Job drawing, mm, ordinate dimensions from the low corner. One solid piece. A direction names the side the tool comes from. Coordinates: 2 decimals unless noted, no trailing zeros. Write each loop counter-clockwise with the first axis right and the second up, starting at its lowest first coordinate (ties: lowest second). Pieces come first, ordered by that corner, then holes. Notation, with made-up numbers: (88, -13.75) - (115, -13.75) arc R26 ccw to (115, 2.25) - close; hole circle Ø3 at (31.25, -23). An arc over 180 degrees is marked (long way). Put each result on its own line as item: value. Start each with the question number.
1. Saw through at B-B, the plane y = 0.5. Write the cut outline in (x, z).
2. Drill centre lines: L1, parallel to Z at x = 1, y = 2; L2, parallel to Y at x = 4.5, z = 4; L3, parallel to Y at x = 4.5, z = 2.5. Where is each one in solid material? Low to high. Write a range as from..to.
3. Saw through at C-C, the plane x = 6.5. Write the cut outline in (y, z).
4. Pull direction Z, two halves, no side cores. Call the marked faces 3, 4, 5 and 6: released by +Z, released by -Z, zero draft, split by the parting line, or undercut.
5. Which spindle directions (+Z, -Z, +X, -X, +Y, -Y) get a long thin tool onto all of the face, cutting with end or side? Do the marked faces 1 and 2. Say none if no direction does.
6. Saw through at A-A, the plane x = 4.5. Write the cut outline in (y, z).
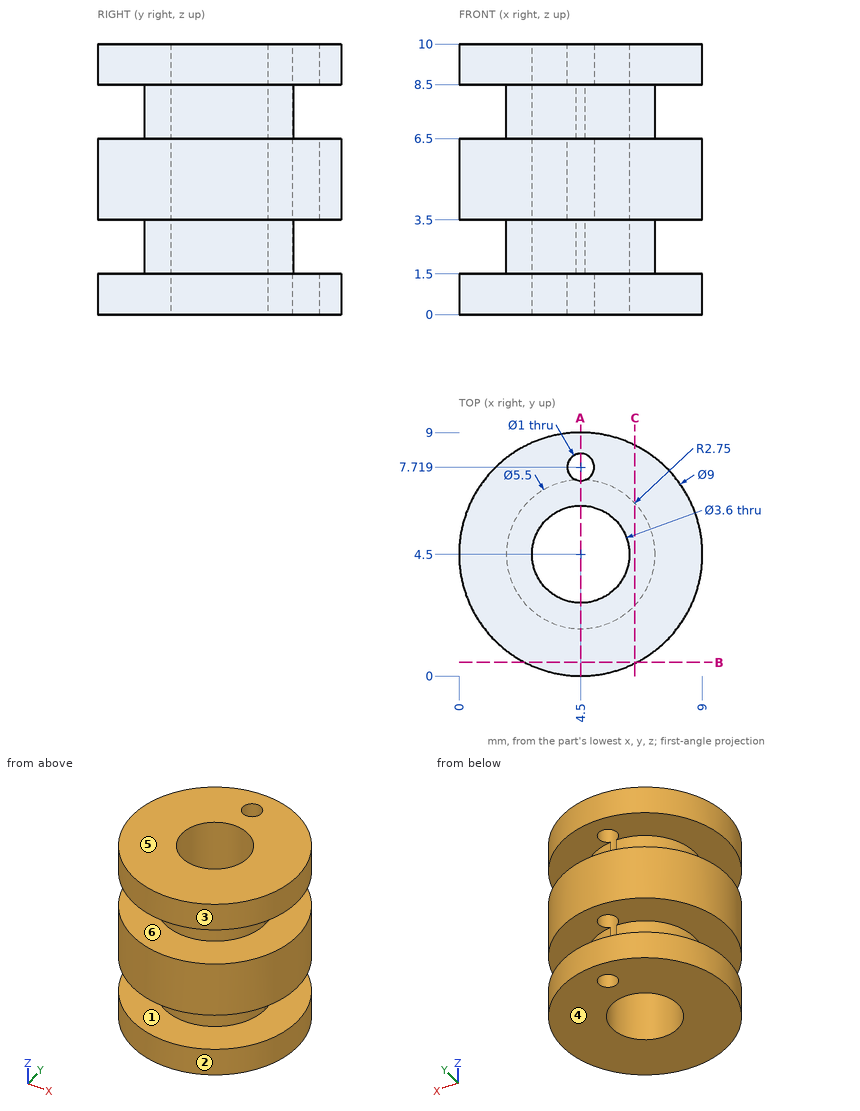
Final values:
1. outline: (2.44, 0) - (6.56, 0) - (6.56, 1.5) - (2.44, 1.5) - close; (2.44, 3.5) - (6.56, 3.5) - (6.56, 6.5) - (2.44, 6.5) - close; (2.44, 8.5) - (6.56, 8.5) - (6.56, 10) - (2.44, 10) - close
2. L1: z = 0..1.5, 3.5..6.5, 8.5..10
2. L2: y = 0..2.7, 6.3..7.22, 8.22..9
2. L3: y = 1.75..2.7, 6.3..7.22
3. outline: (0.47, 0) - (8.53, 0) - (8.53, 1.5) - (6.39, 1.5) - (6.39, 3.5) - (8.53, 3.5) - (8.53, 6.5) - (6.39, 6.5) - (6.39, 8.5) - (8.53, 8.5) - (8.53, 10) - (0.47, 10) - (0.47, 8.5) - (2.61, 8.5) - (2.61, 6.5) - (0.47, 6.5) - (0.47, 3.5) - (2.61, 3.5) - (2.61, 1.5) - (0.47, 1.5) - close
4. face 3: zero draft
4. face 4: released by -Z
4. face 5: released by +Z
4. face 6: undercut
5. face 1: none
5. face 2: +Z, -Z
6. outline: (0, 0) - (2.7, 0) - (2.7, 10) - (0, 10) - (0, 8.5) - (1.75, 8.5) - (1.75, 6.5) - (0, 6.5) - (0, 3.5) - (1.75, 3.5) - (1.75, 1.5) - (0, 1.5) - close; (6.3, 0) - (7.22, 0) - (7.22, 10) - (6.3, 10) - close; (8.22, 0) - (9, 0) - (9, 1.5) - (8.22, 1.5) - close; (8.22, 3.5) - (9, 3.5) - (9, 6.5) - (8.22, 6.5) - close; (8.22, 8.5) - (9, 8.5) - (9, 10) - (8.22, 10) - close
